Work out the finished part from the listing and answer in its coordinate system (mm). A direction names the side the tool comes from. Coordinates: 2 decimals unless noted, no trailing zeros. Loops run counter-clockwise (first coordinate to the right, second up) from the corner with the lowest first, then second, coordinate; pieces in that order, holes last. Notation, with made-up numbers: (-18.5, -28.5) - (33.5, -28.5) arc R33 cw to (33.5, 9.5) - close; hole circle Ø7 at (20, 37). An arc over 180 degrees is marked (long way). Write each question's results on one line, items separated by ' | '. Start each with the question number.
Item 1: Section D-D, the plane z = -8.25 is taken. Write down the section's boundary in (x, y), plus the area to 3 significant figures.
Item 2: A tool of negligible diameter and unlimited length cuts with its end or side. For faces 4 (the face through (-9.55, 8, -5)), 5 (the face through (36, 5, -8.9)), 6 (the face through (-16, 6.3, -5)), from which of +Z, -Z, +X, -X, +Y, -Y can it reach the whole face along a straight path? Write none if from no direction.
Item 3: For a pull along Z with two mould halves and no side action, classify faces 1 (the face through (36, 6.3, 0)), 2 (the face through (39.75, 8, -5)), 3 (the face through (21, 6, -11.5)) as +Z half, -Z half, draft (parallel to the pull), parting line (faces both ways), or undercut.
Item 4: Section A-A, the plane y = 9.5 is taken. Write down the section's boundary in (x, z), plus the area to 3 significant figures.
Item 5: Consider probe 1 along X at (y, z) = (9, -10); probe 2 along X at (y, z) = (7.75, -7.25); probe 3 along Z at (x, y) = (39, 5.5). Determine where each line is inside the solid, lowest interval first. Write a range as [from, to].
Item 6: Each of these flat-tipped pins is pushed along its axis until it touches: pin 1 Ø4.5 at (x, y) = (2.5, 7) entering from -Z; pin 2 Ø0.7 at (y, z) = (5, -10.5) entering from +X; pin 3 Ø5 at (x, z) = (26.5, -14.5) entering from +Y. Where does it stop, or does it pass through?
Item 7: Section C-C, the plane x = 8 is taken. Write down the section's boundary in (y, z).
from build123d import *

# Parameters (mm, degrees)
SKETCH1_W           = 69.9
SKETCH1_H           = 22
BOSS_EXTRUDE1_DEPTH = 1.5
BOSS_EXTRUDE2_START = -1.5
SKETCH2_W           = 10
SKETCH2_H           = 15.3
BOSS_EXTRUDE2_DEPTH = 15.4
BOSS_EXTRUDE3_START = -1.5
SKETCH2_3_W         = 18.6
SKETCH2_3_H         = 15.3
BOSS_EXTRUDE3_DEPTH = 17
SKETCH3_W           = 3
SKETCH3_H           = 3
CUT_EXTRUDE1_DEPTH  = 8
SKETCH4_W           = 3
SKETCH4_H           = 3
CUT_EXTRUDE2_DEPTH  = 8
BOSS_EXTRUDE5_START = -1.5
SKETCH5_W           = 4.9
SKETCH5_H           = 2.2
BOSS_EXTRUDE5_DEPTH = 10.7
BOSS_EXTRUDE6_START = -1.5
SKETCH5_3_W         = 6.1
SKETCH5_3_H         = 3.9
BOSS_EXTRUDE6_DEPTH = 5.4
SKETCH6_W           = 53
SKETCH6_H           = 14.6
BOSS_EXTRUDE7_DEPTH = 1


with BuildPart() as part:
    # Sketch1 → Boss-Extrude1 (new body)
    with BuildSketch(Plane(origin=(0, 0, 0), x_dir=(1, 0, 0), z_dir=(0, 1, 0))):
        with Locations((9.6, 7.6)):
            Rectangle(SKETCH1_W, SKETCH1_H)
    extrude(amount=BOSS_EXTRUDE1_DEPTH)

    # Sketch2 → Boss-Extrude2 (add)
    with BuildSketch(Plane(origin=(0, 1.5, 0), x_dir=(1, 0, 0), z_dir=(0, 1, 0)).offset(BOSS_EXTRUDE2_START)):
        with Locations((-14.55, 5.25)):
            Rectangle(SKETCH2_W, SKETCH2_H)
        with Locations((34.75, 5.15)):
            Rectangle(SKETCH2_W, SKETCH2_H)
    extrude(amount=BOSS_EXTRUDE2_DEPTH)

    # Sketch2<3> → Boss-Extrude3 (add)
    with BuildSketch(Plane(origin=(0, 1.5, 0), x_dir=(1, 0, 0), z_dir=(0, 1, 0)).offset(BOSS_EXTRUDE3_START)):
        with Locations((0.75, 5.15)):
            Rectangle(SKETCH2_3_W, SKETCH2_3_H)
    extrude(amount=BOSS_EXTRUDE3_DEPTH)

    # Sketch3 → Cut-Extrude1 (cut)
    with BuildSketch(Plane.ZY.offset(19.55)):
        with Locations((-10.4, 4.8)):
            Rectangle(SKETCH3_W, SKETCH3_H)
        with Locations((-5.25, 4.8)):
            Rectangle(SKETCH3_W, SKETCH3_H)
        with Locations((-0.1, 4.8)):
            Rectangle(SKETCH3_W, SKETCH3_H)
    extrude(amount=-CUT_EXTRUDE1_DEPTH, mode=Mode.SUBTRACT)

    # Sketch4 → Cut-Extrude2 (cut)
    with BuildSketch(Plane(origin=(39.75, 0, 0), x_dir=(0, 0, -1), z_dir=(1, 0, 0))):
        with Locations((10.4, 4.8)):
            Rectangle(SKETCH4_W, SKETCH4_H)
        with Locations((5.25, 4.8)):
            Rectangle(SKETCH4_W, SKETCH4_H)
        with Locations((0.1, 4.8)):
            Rectangle(SKETCH4_W, SKETCH4_H)
    extrude(amount=-CUT_EXTRUDE2_DEPTH, mode=Mode.SUBTRACT)

    # Sketch5 → Boss-Extrude5 (add)
    with BuildSketch(Plane(origin=(0, 1.5, 0), x_dir=(1, 0, 0), z_dir=(0, 1, 0)).offset(BOSS_EXTRUDE5_START)):
        with Locations((21.3, 10.4)):
            Rectangle(SKETCH5_W, SKETCH5_H)
        with Locations((21.3, -1.1)):
            Rectangle(SKETCH5_W, SKETCH5_H)
    extrude(amount=BOSS_EXTRUDE5_DEPTH)

    # Sketch5<3> → Boss-Extrude6 (add)
    with BuildSketch(Plane(origin=(0, 1.5, 0), x_dir=(1, 0, 0), z_dir=(0, 1, 0)).offset(BOSS_EXTRUDE6_START)):
        with Locations((21.5, 4.65)):
            Rectangle(SKETCH5_3_W, SKETCH5_3_H)
    extrude(amount=BOSS_EXTRUDE6_DEPTH)

    # Sketch6 → Boss-Extrude7 (add)
    with BuildSketch(Plane.XZ):
        with Locations((9.45, -5.1)):
            Rectangle(SKETCH6_W, SKETCH6_H)
    extrude(amount=BOSS_EXTRUDE7_DEPTH)


solid = part.part
Answer key:
1) outline: (-25.35, 0) - (-17.05, 0) - (-17.05, -1) - (35.95, -1) - (35.95, 0) - (44.55, 0) - (44.55, 1.5) - (39.75, 1.5) - (39.75, 15.4) - (29.75, 15.4) - (29.75, 1.5) - (10.05, 1.5) - (10.05, 17) - (-8.55, 17) - (-8.55, 1.5) - (-9.55, 1.5) - (-9.55, 15.4) - (-19.55, 15.4) - (-19.55, 1.5) - (-25.35, 1.5) - close | area: 724 mm^2
2) face 4: +Z, -Z, +Y | face 5: +X | face 6: -X
3) face 1: undercut | face 2: draft | face 3: -Z half
4) outline: (-19.55, -12.9) - (-9.55, -12.9) - (-9.55, 2.4) - (-19.55, 2.4) - close; (-8.55, -12.8) - (10.05, -12.8) - (10.05, 2.5) - (-8.55, 2.5) - close; (18.85, -11.5) - (23.75, -11.5) - (23.75, -9.3) - (18.85, -9.3) - close; (18.85, 0) - (23.75, 0) - (23.75, 2.2) - (18.85, 2.2) - close; (29.75, -12.8) - (39.75, -12.8) - (39.75, 2.5) - (29.75, 2.5) - close | area: 612 mm^2
5) probe 1: x = [-19.55, -9.55], [-8.55, 10.05], [18.85, 23.75], [29.75, 39.75] | probe 2: x = [-19.55, -9.55], [-8.55, 10.05], [29.75, 39.75] | probe 3: z = [-12.8, -11.9], [-8.9, -6.75], [-3.75, -1.6], [1.4, 2.5]
6) pin 1: stops at z = -12.8 | pin 2: stops at x = 31.75 | pin 3: stops at y = 1.5
7) outline: (-1, -12.4) - (0, -12.4) - (0, -18.6) - (1.5, -18.6) - (1.5, -12.8) - (17, -12.8) - (17, 2.5) - (1.5, 2.5) - (1.5, 3.4) - (0, 3.4) - (0, 2.2) - (-1, 2.2) - close
